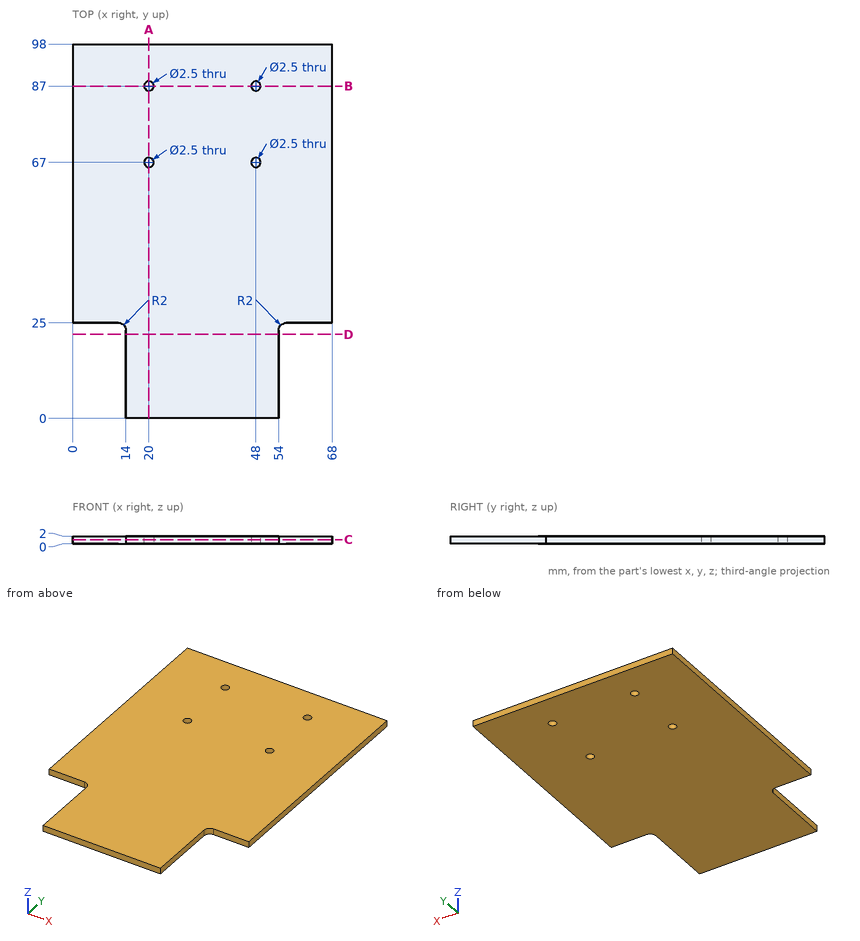
Could you check a few things on this drawing? It's one solid part, dimensions in mm from its lowest x, y, z. Coordinates: 2 decimals unless noted, no trailing zeros. Order: outer loops, then holes, each group sorted by start corner. A loop starts at its lowest first (then second) coordinate and runs counter-clockwise, first axis right, second up. Notation, with made-up numbers: (4, 45) -> (16, 45) arc R19 cw to (16, 71) -> close; hole circle Ø9 at (50.5, -1). An arc over 180 degrees is marked (long way). One line per item, written item: value. Start each with the question number.
1) Imagine slicing it at A-A on x = 20. List the corners of the cut face in (y, z) for me.
2) Imagine slicing it at C-C on z = 1.15. List the corners of the cut face in (x, y) for me, plus the area to 3 significant figures.
3) I'm going to push flat-ended pins straight in: pin 1 (1.5 mm diameter, centred on x = 20, y = 87, fed in from -Z); pin 2 (1 mm diameter, centred on x = 5.5, z = 1.5, fed in from -Y). Where does each tip first touch, or does it pass through?
4) If I drill on L1, parallel to Y at x = 48, z = 1.4; L2, parallel to X at y = 87, z = 0.45; L3, parallel to Y at x = 48.5, z = 1.75, over which ranges is the centre line in solid material (lowest first)? Write a range as [from, to].
5) Imagine slicing it at D-D on y = 22. List the corners of the cut face in (x, z) for me.
6) Imagine slicing it at B-B on y = 87. List the corners of the cut face in (x, z) for me.
Answer list:
1. outline: (0, 0) -> (65.75, 0) -> (65.75, 2) -> (0, 2) -> close; (68.25, 0) -> (85.75, 0) -> (85.75, 2) -> (68.25, 2) -> close; (88.25, 0) -> (98, 0) -> (98, 2) -> (88.25, 2) -> close
2. outline: (0, 25) -> (12, 25) arc R2 cw to (14, 23) -> (14, 0) -> (54, 0) -> (54, 23) arc R2 cw to (56, 25) -> (68, 25) -> (68, 98) -> (0, 98) -> close; hole circle Ø2.5 at (20, 67); hole circle Ø2.5 at (20, 87); hole circle Ø2.5 at (48, 67); hole circle Ø2.5 at (48, 87)
2. area: 5,950 mm2
3. pin 1: passes through
3. pin 2: stops at y = 25
4. L1: y = [0, 65.75], [68.25, 85.75], [88.25, 98]
4. L2: x = [0, 18.75], [21.25, 46.75], [49.25, 68]
4. L3: y = [0, 65.85], [68.15, 85.85], [88.15, 98]
5. outline: (14, 0) -> (54, 0) -> (54, 2) -> (14, 2) -> close
6. outline: (0, 0) -> (18.75, 0) -> (18.75, 2) -> (0, 2) -> close; (21.25, 0) -> (46.75, 0) -> (46.75, 2) -> (21.25, 2) -> close; (49.25, 0) -> (68, 0) -> (68, 2) -> (49.25, 2) -> close
